Read the model definition and answer for the solid it produces. Units are mm, in the model's axes. Give positions to 0.01 mm unless a question says otherwise; leave off trailing zeros. Order: outer loops, then holes, each group sorted by start corner. A loop starts at its lowest first (then second) coordinate and runs counter-clockwise, first axis right, second up.
Item 1: A cutting plane is placed at D-D (y = -23). Write down the section's boundary in (x, z).
Item 2: Given pin 1 Ø1.5 at (y, z) = (-20.5, -2.5) entering from -X; pin 2 Ø1 at (y, z) = (-53, -1) entering from +X; pin 3 Ø6 at (x, y) = (45, -75) entering from +Z; pin 4 Ø2.5 at (x, z) = (-60, -1.5) entering from -Y, each flat-ended and moving along its own axis, determine where each tip first touches the part or whether it passes through.
Item 3: Find the intervals of material crossed by line 1 along X through (y, z) = (-22.5, -3.9); line 2 along Y through (x, z) = (-53, -4.1); line 3 along Y through (x, z) = (-62, -0.7), in increasing order.
Item 4: A cutting plane is placed at C-C (x = 59). Write down the section's boundary in (y, z).
Item 5: A cutting plane is placed at B-B (z = -1.05). Write down the section's boundary in (x, y), plus the area to 3 significant figures.
Item 6: A cutting plane is placed at A-A (x = -57.5). Write down the section's boundary in (y, z).
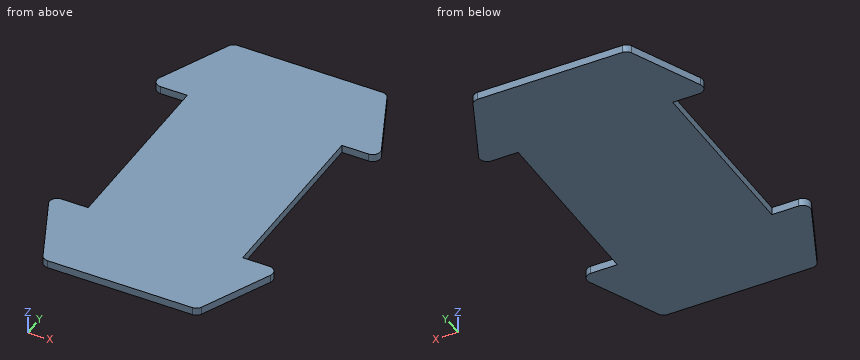
from build123d import *

# Parameters (mm, degrees)
BOSS_EXTRUDE1_DEPTH = 5
FILLET2_R           = 5


with BuildPart() as part:
    # Sketch3 → Boss-Extrude1 (new body)
    with BuildSketch(Plane.XY):
        Polygon((50, 115), (-50, 115), (-75, 60), (-50, 60), (-50, -60), (-75, -60), (-50, -115), (50, -115), (75, -60), (50, -60), (50, 60), (75, 60), align=None)
    extrude(amount=-BOSS_EXTRUDE1_DEPTH)

    # Fillet2
    fillet2_edges = [part.edges().sort_by_distance(p)[0] for p in [
        (-50, 115, -2.5),
        (50, 115, -2.5),
        (75, 60, -2.5),
        (75, -60, -2.5),
        (50, -115, -2.5),
        (-50, -115, -2.5),
        (-75, -60, -2.5),
        (-75, 60, -2.5),
    ]]
    fillet(fillet2_edges, radius=FILLET2_R)


solid = part.part
Response values:
1. outline: (-50, -5) - (50, -5) - (50, 0) - (-50, 0) - close
2. pin 1: stops at x = -50
2. pin 2: stops at x = 50
2. pin 3: stops at z = 0
2. pin 4: stops at y = -95.75
3. line 1: x = -50 to 50
3. line 2: y = -108.4 to -60, 60 to 108.4
3. line 3: y = -88.6 to -60, 60 to 88.6
4. outline: (-95.2, -5) - (-60, -5) - (-60, 0) - (-95.2, 0) - close; (60, -5) - (95.2, -5) - (95.2, 0) - (60, 0) - close
5. outline: (-71.79, -67.07) - (-51.33, -112.07) arc R5 ccw to (-46.78, -115) - (46.78, -115) arc R5 ccw to (51.33, -112.07) - (71.79, -67.07) arc R5 ccw to (67.23, -60) - (50, -60) - (50, 60) - (67.23, 60) arc R5 ccw to (71.79, 67.07) - (51.33, 112.07) arc R5 ccw to (46.78, 115) - (-46.78, 115) arc R5 ccw to (-51.33, 112.07) - (-71.79, 67.07) arc R5 ccw to (-67.23, 60) - (-50, 60) - (-50, -60) - (-67.23, -60) arc R5 ccw to start
5. area: 25,700 mm2
6. outline: (-98.5, -5) - (-60, -5) - (-60, 0) - (-98.5, 0) - close; (60, -5) - (98.5, -5) - (98.5, 0) - (60, 0) - close
